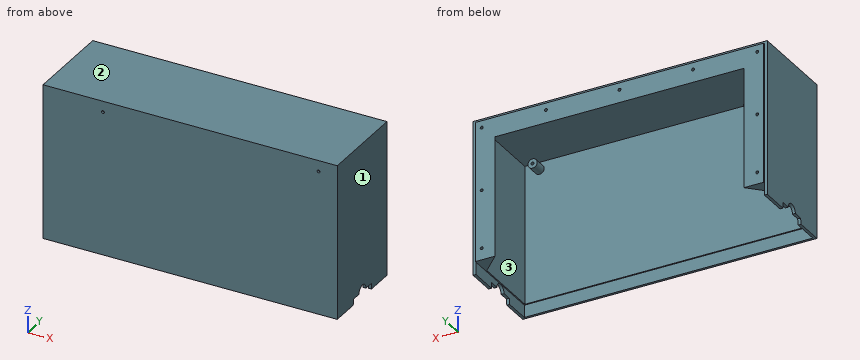
from build123d import *

# Parameters (mm, degrees)
SKETCH1_W               = 247.42
SKETCH1_H               = 129.49
SKETCH1_R               = 4
SKETCH1_W_2             = 2.5
SKETCH1_R_2             = 1.25
BOSS_EXTRUDE1_DEPTH     = 2
BOSS_EXTRUDE2_START     = 2
SKETCH1_6_R             = 4
SKETCH1_6_R_2           = 1.25
BOSS_EXTRUDE2_DEPTH     = 11.7
BOSS_EXTRUDE3_START     = 2
SKETCH1_7_W             = 2.5
SKETCH1_7_H             = 129.49
BOSS_EXTRUDE3_DEPTH     = 75.64
SKETCH2_W               = 247.42
SKETCH2_H               = 118.92
BOSS_EXTRUDE4_DEPTH     = 1
SKETCH3_W               = 118.92
SKETCH3_H               = 74.64
BOSS_EXTRUDE5_DEPTH     = 1
SKETCH4_W               = 118.92
SKETCH4_H               = 74.64
BOSS_EXTRUDE6_DEPTH     = 1
CUT_EXTRUDE1_DEPTH      = 296.461378356
CUT_EXTRUDE1_DEPTH_BACK = 296.461378356
BOSS_EXTRUDE7_DEPTH     = 118.92
BOSS_EXTRUDE8_REACH     = 297.461
CUT_EXTRUDE2_REACH      = 295.328
SKETCH8_R               = 1.25
SKETCH9_W               = 247.42
SKETCH9_H               = 2
CUT_EXTRUDE3_DEPTH      = 1


with BuildPart() as part:
    # Sketch1 → Boss-Extrude1 (new body)
    # profile 1 of 6: a face of its own
    with BuildSketch(Plane(origin=(0, 0, 0), x_dir=(1, 0, 0), z_dir=(0, 1, 0))):
        with Locations((123.71, -64.745)):
            Rectangle(SKETCH1_W, SKETCH1_H)
        with Locations((48.85, -123.16)):
            Circle(SKETCH1_R, mode=Mode.SUBTRACT)
        with Locations((233.87, -123.16)):
            Circle(SKETCH1_R, mode=Mode.SUBTRACT)
    # profile 2 of 6: a face of its own
    with BuildSketch(Plane(origin=(0, 0, 0), x_dir=(1, 0, 0), z_dir=(0, 1, 0))):
        with Locations((-1.25, -64.745)):
            Rectangle(SKETCH1_W_2, SKETCH1_H)
    # profile 3 of 6: a face of its own
    with BuildSketch(Plane(origin=(0, 0, 0), x_dir=(1, 0, 0), z_dir=(0, 1, 0))):
        Polygon((249.92, -129.49), (249.92, -132.49), (-2.5, -132.49), (-2.5, -129.49), (0, -129.49), (247.42, -129.49), align=None)
    # profile 4 of 6: a face of its own
    with BuildSketch(Plane(origin=(0, 0, 0), x_dir=(1, 0, 0), z_dir=(0, 1, 0))):
        with Locations((248.67, -64.745)):
            Rectangle(SKETCH1_W_2, SKETCH1_H)
    # profile 5 of 6: a face of its own
    with BuildSketch(Plane(origin=(0, 0, 0), x_dir=(1, 0, 0), z_dir=(0, 1, 0))):
        with Locations((233.87, -123.16)):
            Circle(SKETCH1_R)
        with Locations(Location((233.87, -123.16, 0), (0, 0, 270))):
            Circle(SKETCH1_R_2, mode=Mode.SUBTRACT)
    # profile 6 of 6: a face of its own
    with BuildSketch(Plane(origin=(0, 0, 0), x_dir=(1, 0, 0), z_dir=(0, 1, 0))):
        with Locations((48.85, -123.16)):
            Circle(SKETCH1_R)
        with Locations(Location((48.85, -123.16, 0), (0, 0, 270))):
            Circle(SKETCH1_R_2, mode=Mode.SUBTRACT)
    extrude(amount=BOSS_EXTRUDE1_DEPTH)

    # Sketch1<6> → Boss-Extrude2 (add)
    # profile 1 of 2: a face of its own
    with BuildSketch(Plane(origin=(0, 0, 0), x_dir=(1, 0, 0), z_dir=(0, 1, 0)).offset(BOSS_EXTRUDE2_START)):
        with Locations(Location((48.85, -123.16, 0), (0, 0, 270))):
            Circle(SKETCH1_6_R)
        with Locations(Location((48.85, -123.16, 0), (0, 0, 270))):
            Circle(SKETCH1_6_R_2, mode=Mode.SUBTRACT)
    # profile 2 of 2: a face of its own
    with BuildSketch(Plane(origin=(0, 0, 0), x_dir=(1, 0, 0), z_dir=(0, 1, 0)).offset(BOSS_EXTRUDE2_START)):
        with Locations(Location((233.87, -123.16, 0), (0, 0, 270))):
            Circle(SKETCH1_6_R)
        with Locations(Location((233.87, -123.16, 0), (0, 0, 270))):
            Circle(SKETCH1_6_R_2, mode=Mode.SUBTRACT)
    extrude(amount=BOSS_EXTRUDE2_DEPTH)

    # Sketch1<7> → Boss-Extrude3 (add)
    with BuildSketch(Plane(origin=(0, 0, 0), x_dir=(1, 0, 0), z_dir=(0, 1, 0)).offset(BOSS_EXTRUDE3_START)):
        with Locations((-1.25, -64.745)):
            Rectangle(SKETCH1_7_W, SKETCH1_7_H)
        Polygon((249.92, -129.49), (249.92, -132.49), (-2.5, -132.49), (-2.5, -129.49), (0, -129.49), (247.42, -129.49), align=None)
        with Locations((248.67, -64.745)):
            Rectangle(SKETCH1_7_W, SKETCH1_7_H)
    extrude(amount=BOSS_EXTRUDE3_DEPTH)

    # Sketch2 → Boss-Extrude4 (add)
    with BuildSketch(Plane(origin=(0, 2, 0), x_dir=(1, 0, 0), z_dir=(0, 1, 0))):
        with Locations((123.71, -70.03)):
            Rectangle(SKETCH2_W, SKETCH2_H)
    extrude(amount=BOSS_EXTRUDE4_DEPTH)

    # Sketch3 → Boss-Extrude5 (add)
    with BuildSketch(Plane(origin=(0, 0, 0), x_dir=(0, 0, -1), z_dir=(1, 0, 0))):
        with Locations((-70.03, 40.32)):
            Rectangle(SKETCH3_W, SKETCH3_H)
    extrude(amount=BOSS_EXTRUDE5_DEPTH)

    # Sketch4 → Boss-Extrude6 (add)
    with BuildSketch(Plane.ZY.offset(-247.42)):
        with Locations((70.03, 40.32)):
            Rectangle(SKETCH4_W, SKETCH4_H)
    extrude(amount=BOSS_EXTRUDE6_DEPTH)

    # Sketch5 → Cut-Extrude1 (cut, two sides: drawn at the far end of the back side and taken through both)
    with BuildSketch(Plane(origin=(249.92, 0, 0), x_dir=(0, 0, -1), z_dir=(1, 0, 0)).offset(-CUT_EXTRUDE1_DEPTH_BACK)):
        Polygon((-5, 25.285), (0, 24.52), (0, 52.64), (-5, 52.355), (-5, 44.245), (-5, 33.395), align=None)
        with BuildLine():
            ThreePointArc((-5, 44.245), (-10.425, 38.82), (-5, 33.395))
            Line((-5, 33.395), (-5, 44.245))
        make_face()
    extrude(amount=CUT_EXTRUDE1_DEPTH + CUT_EXTRUDE1_DEPTH_BACK, mode=Mode.SUBTRACT)

    # Sketch6 → Boss-Extrude7 (add)
    with BuildSketch(Plane(origin=(0, 0, 129.49), x_dir=(-1, 0, 0), z_dir=(0, 0, -1))):
        Polygon((-246.42, 77.64), (-230.42, 77.64), (-246.42, 61.64), align=None)
        Polygon((-1, 77.64), (-17, 77.64), (-1, 61.64), align=None)
    extrude(amount=BOSS_EXTRUDE7_DEPTH)

    # Boss-Extrude8: up to this plane
    boss_extrude8_end = Plane(origin=(17, 77.64, -12.057416998), z_dir=(-0.7071067811865476, 0.7071067811865476, 0))
    # Sketch7 → Boss-Extrude8 (add, up to the surface)
    with BuildSketch(Plane(origin=(249.92, 0, 0), x_dir=(0, 0, -1), z_dir=(1, 0, 0)), mode=Mode.PRIVATE) as boss_extrude8_sk1:
        Polygon((-132.49, 77.64), (-132.49, 61.64), (-129.49, 61.64), (-113.49, 77.64), align=None)
    boss_extrude8_tool1 = split(extrude(boss_extrude8_sk1.sketch, amount=-BOSS_EXTRUDE8_REACH, mode=Mode.PRIVATE), bisect_by=boss_extrude8_end, keep=Keep.BOTH, mode=Mode.PRIVATE)
    add(boss_extrude8_tool1.solids().sort_by_distance((249.92, 71.579394, 126.020303))[0])

    # Sketch8 → Cut-Extrude2 (cut, up to next)
    with BuildSketch(Plane(origin=(0, 77.64, 0), x_dir=(1, 0, 0), z_dir=(0, 1, 0)), mode=Mode.PRIVATE) as cut_extrude2_sk1:
        with Locations(Location((5.5, -124.49, 0), (0, 0, 270))):
            Circle(SKETCH8_R)
    cut_extrude2_tool1 = extrude(cut_extrude2_sk1.sketch, amount=-CUT_EXTRUDE2_REACH, mode=Mode.PRIVATE) & part.part
    # Sketch8 → Cut-Extrude2 (cut, up to next)
    with BuildSketch(Plane(origin=(0, 77.64, 0), x_dir=(1, 0, 0), z_dir=(0, 1, 0)), mode=Mode.PRIVATE) as cut_extrude2_sk2:
        with Locations(Location((241.92, -124.49, 0), (0, 0, 270))):
            Circle(SKETCH8_R)
    cut_extrude2_tool2 = extrude(cut_extrude2_sk2.sketch, amount=-CUT_EXTRUDE2_REACH, mode=Mode.PRIVATE) & part.part
    # Sketch8 → Cut-Extrude2 (cut, up to next)
    with BuildSketch(Plane(origin=(0, 77.64, 0), x_dir=(1, 0, 0), z_dir=(0, 1, 0)), mode=Mode.PRIVATE) as cut_extrude2_sk3:
        with Locations(Location((60.605, -124.49, 0), (0, 0, 270))):
            Circle(SKETCH8_R)
    cut_extrude2_tool3 = extrude(cut_extrude2_sk3.sketch, amount=-CUT_EXTRUDE2_REACH, mode=Mode.PRIVATE) & part.part
    # Sketch8 → Cut-Extrude2 (cut, up to next)
    with BuildSketch(Plane(origin=(0, 77.64, 0), x_dir=(1, 0, 0), z_dir=(0, 1, 0)), mode=Mode.PRIVATE) as cut_extrude2_sk4:
        with Locations(Location((186.815, -124.49, 0), (0, 0, 270))):
            Circle(SKETCH8_R)
    cut_extrude2_tool4 = extrude(cut_extrude2_sk4.sketch, amount=-CUT_EXTRUDE2_REACH, mode=Mode.PRIVATE) & part.part
    # Sketch8 → Cut-Extrude2 (cut, up to next)
    with BuildSketch(Plane(origin=(0, 77.64, 0), x_dir=(1, 0, 0), z_dir=(0, 1, 0)), mode=Mode.PRIVATE) as cut_extrude2_sk5:
        with Locations(Location((123.71, -124.49, 0), (0, 0, 270))):
            Circle(SKETCH8_R)
    cut_extrude2_tool5 = extrude(cut_extrude2_sk5.sketch, amount=-CUT_EXTRUDE2_REACH, mode=Mode.PRIVATE) & part.part
    # Sketch8 → Cut-Extrude2 (cut, up to next)
    with BuildSketch(Plane(origin=(0, 77.64, 0), x_dir=(1, 0, 0), z_dir=(0, 1, 0)), mode=Mode.PRIVATE) as cut_extrude2_sk6:
        with Locations(Location((5.5, -70.57, 0), (0, 0, 270))):
            Circle(SKETCH8_R)
    cut_extrude2_tool6 = extrude(cut_extrude2_sk6.sketch, amount=-CUT_EXTRUDE2_REACH, mode=Mode.PRIVATE) & part.part
    # Sketch8 → Cut-Extrude2 (cut, up to next)
    with BuildSketch(Plane(origin=(0, 77.64, 0), x_dir=(1, 0, 0), z_dir=(0, 1, 0)), mode=Mode.PRIVATE) as cut_extrude2_sk7:
        with Locations(Location((5.5, -20.57, 0), (0, 0, 270))):
            Circle(SKETCH8_R)
    cut_extrude2_tool7 = extrude(cut_extrude2_sk7.sketch, amount=-CUT_EXTRUDE2_REACH, mode=Mode.PRIVATE) & part.part
    # Sketch8 → Cut-Extrude2 (cut, up to next)
    with BuildSketch(Plane(origin=(0, 77.64, 0), x_dir=(1, 0, 0), z_dir=(0, 1, 0)), mode=Mode.PRIVATE) as cut_extrude2_sk8:
        with Locations(Location((241.92, -20.57, 0), (0, 0, 270))):
            Circle(SKETCH8_R)
    cut_extrude2_tool8 = extrude(cut_extrude2_sk8.sketch, amount=-CUT_EXTRUDE2_REACH, mode=Mode.PRIVATE) & part.part
    # Sketch8 → Cut-Extrude2 (cut, up to next)
    with BuildSketch(Plane(origin=(0, 77.64, 0), x_dir=(1, 0, 0), z_dir=(0, 1, 0)), mode=Mode.PRIVATE) as cut_extrude2_sk9:
        with Locations(Location((241.92, -70.57, 0), (0, 0, 270))):
            Circle(SKETCH8_R)
    cut_extrude2_tool9 = extrude(cut_extrude2_sk9.sketch, amount=-CUT_EXTRUDE2_REACH, mode=Mode.PRIVATE) & part.part
    add(cut_extrude2_tool1.solids().sort_by_distance((5.5, 77.64, 124.49))[0], mode=Mode.SUBTRACT)
    add(cut_extrude2_tool2.solids().sort_by_distance((241.92, 77.64, 124.49))[0], mode=Mode.SUBTRACT)
    add(cut_extrude2_tool3.solids().sort_by_distance((60.605, 77.64, 124.49))[0], mode=Mode.SUBTRACT)
    add(cut_extrude2_tool4.solids().sort_by_distance((186.815, 77.64, 124.49))[0], mode=Mode.SUBTRACT)
    add(cut_extrude2_tool5.solids().sort_by_distance((123.71, 77.64, 124.49))[0], mode=Mode.SUBTRACT)
    add(cut_extrude2_tool6.solids().sort_by_distance((5.5, 77.64, 70.57))[0], mode=Mode.SUBTRACT)
    add(cut_extrude2_tool7.solids().sort_by_distance((5.5, 77.64, 20.57))[0], mode=Mode.SUBTRACT)
    add(cut_extrude2_tool8.solids().sort_by_distance((241.92, 77.64, 20.57))[0], mode=Mode.SUBTRACT)
    add(cut_extrude2_tool9.solids().sort_by_distance((241.92, 77.64, 70.57))[0], mode=Mode.SUBTRACT)

    # Sketch9 → Cut-Extrude3 (cut)
    with BuildSketch(Plane(origin=(0, 77.64, 0), x_dir=(1, 0, 0), z_dir=(0, 1, 0))):
        Polygon((0, 0), (-2.5, 0), (-2.5, -132.49), (0, -132.49), (0, -130.49), align=None)
        with Locations((123.71, -131.49)):
            Rectangle(SKETCH9_W, SKETCH9_H)
        Polygon((247.42, 0), (247.42, -130.49), (247.42, -132.49), (249.92, -132.49), (249.92, 0), align=None)
    extrude(amount=-CUT_EXTRUDE3_DEPTH, mode=Mode.SUBTRACT)


solid = part.part
The listing builds one solid part. Answer for the finished solid, in the listing's coordinates (mm). Face numbers are marked on the shaded views. Give positions to 0.01 mm unless a question says otherwise; leave off trailing zeros. Write each loop counter-clockwise with the first axis right and the second up, starting at its lowest first coordinate (ties: lowest second). Pieces come first, ordered by that corner, then holes.
1) Section D-D (z = 94) is taken. Write down the section's boundary in (x, y).
2) Find the intervals of material crossed by L1, parallel to X at y = 68, z = 124.49 (3 decimals); L2, parallel to X at y = 6.5, z = 123.16; L3, parallel to Z at x = 241, y = 69, in increasing order.
3) Section B-B (x = 21) is taken. Write down the section's boundary in (y, z).
4) Section C-C (y = 38.82) is taken. Write down the section's boundary in (x, z) (3 decimals), and give its area (3 significant figures).
5) Section A-A (y = 9) is taken. Write down the section's boundary in (x, z), and give its area (3 significant figures).
6) Given P1, Ø3, axis at x = 23, y = 56, coming from the -Z side; P2, Ø3, axis at x = 150, z = 94.5, coming from the +Y side; P3, Ø1.2, axis at x = -2, y = 50, coming from the -Z side, each flat-ended and moving along its own axis, determine where each tip first touches the part or whether it passes through.
7) For a pull along X with two mould halves and no side action, classify the marked faces 1, 2 and 3 as pulls with the +X half, pulls with the -X half, needs draft (parallel to the pull), parting line crosses it, or undercut.
Response:
1. outline: (-2.5, 0) - (249.92, 0) - (249.92, 76.64) - (247.42, 76.64) - (247.42, 77.64) - (230.42, 77.64) - (246.42, 61.64) - (246.42, 3) - (1, 3) - (1, 61.64) - (17, 77.64) - (0, 77.64) - (0, 76.64) - (-2.5, 76.64) - close
2. L1: x = -2.5 to 4.25, 6.75 to 59.355, 61.855 to 122.46, 124.96 to 185.565, 188.065 to 240.67, 243.17 to 249.92
2. L2: x = -2.5 to 1, 44.85 to 47.6, 50.1 to 52.85, 229.87 to 232.62, 235.12 to 237.87, 246.42 to 249.92
2. L3: z = 10.57 to 19.72, 21.42 to 69.72, 71.42 to 123.64, 125.34 to 132.49
3. outline: (0, 0) - (2, 0) - (2, 10.57) - (3, 10.57) - (3, 129.49) - (61.64, 129.49) - (77.64, 113.49) - (77.64, 130.49) - (76.64, 130.49) - (76.64, 132.49) - (0, 132.49) - close
4. outline: (-2.5, 10.425) - (0, 10.425) - (0, 10.57) - (1, 10.57) - (1, 129.49) - (246.42, 129.49) - (246.42, 10.57) - (247.42, 10.57) - (247.42, 10.425) - (249.92, 10.425) - (249.92, 132.49) - (-2.5, 132.49) - close
4. area: 1,590 mm2
5. outline: (-2.5, 0) - (0, 0) - (0, 10.57) - (1, 10.57) - (1, 129.49) - (246.42, 129.49) - (246.42, 10.57) - (247.42, 10.57) - (247.42, 0) - (249.92, 0) - (249.92, 132.49) - (-2.5, 132.49) - close; circle Ø8 at (48.85, 123.16); circle Ø8 at (233.87, 123.16); hole circle Ø2.5 at (48.85, 123.16); hole circle Ø2.5 at (233.87, 123.16)
5. area: 1,730 mm2
6. P1: stops at z = 129.49
6. P2: stops at y = 3
6. P3: stops at z = 5
7. face 1: pulls with the +X half
7. face 2: needs draft
7. face 3: undercut
